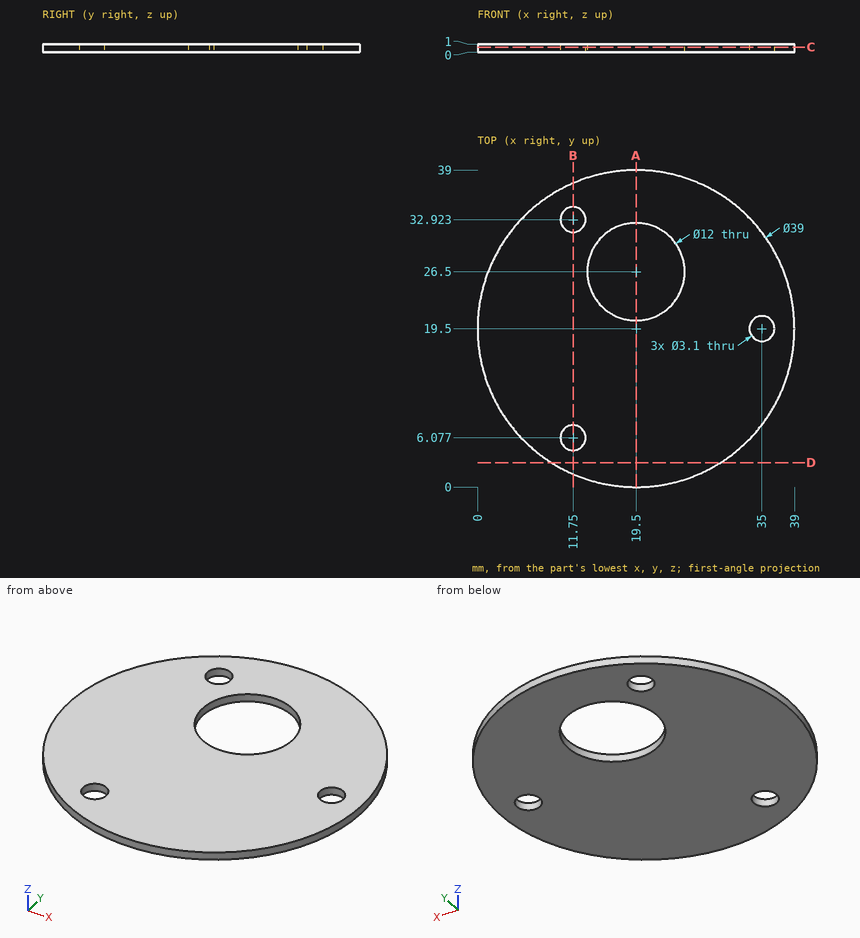
Study the drawing (mm; zero at the part's minimum x, y, z) and answer. Give positions to 0.01 mm unless a question says otherwise; leave off trailing zeros. Write each loop counter-clockwise with the first axis right and the second up, starting at its lowest first coordinate (ties: lowest second). Pieces come first, ordered by that corner, then holes.
Item 1: Section D-D, the plane y = 3 is taken. Write down the section's boundary in (x, z), plus the area to 3 significant figures.
Item 2: Find the intervals of material crossed by line 1 along Y through (x, z) = (11.75, 0.85) (1 decimal); line 2 along Y through (x, z) = (19.5, 0.6); line 3 along Y through (x, z) = (12.5, 0.7), in increasing order.
Item 3: Section C-C, the plane z = 0.6 is taken. Write down the section's boundary in (x, y).
Item 4: Section B-B, the plane x = 11.75 is taken. Write down the section's boundary in (y, z).
Item 5: Section A-A, the plane x = 19.5 is taken. Write down the section's boundary in (y, z), plus the area to 3 significant figures.
Item 6: A flat-ended cylindrical pin translates along its axis: P1, Ø2.5, axis at x = 11.75, y = 32.92, coming from the +Z side. Find the tip coordinate at first contact, or state that the pin passes through.
Completed:
1. outline: (9.11, 0) - (29.89, 0) - (29.89, 1) - (9.11, 1) - close
1. area: 20.8 mm2
2. line 1: y = 1.6 to 4.5, 7.6 to 31.4, 34.5 to 37.4
2. line 2: y = 0 to 20.5, 32.5 to 39
2. line 3: y = 1.3 to 4.72, 7.43 to 31.57, 34.28 to 37.7
3. outline: circle Ø39 at (19.5, 19.5); hole circle Ø3.1 at (11.75, 6.08); hole circle Ø3.1 at (11.75, 32.92); hole circle Ø12 at (19.5, 26.5); hole circle Ø3.1 at (35, 19.5)
4. outline: (1.61, 0) - (4.53, 0) - (4.53, 1) - (1.61, 1) - close; (7.63, 0) - (31.37, 0) - (31.37, 1) - (7.63, 1) - close; (34.47, 0) - (37.39, 0) - (37.39, 1) - (34.47, 1) - close
5. outline: (0, 0) - (20.5, 0) - (20.5, 1) - (0, 1) - close; (32.5, 0) - (39, 0) - (39, 1) - (32.5, 1) - close
5. area: 27.0 mm2
6. P1: passes through
